from build123d import *
from build123d.topology import SkipClean

# Parameters (mm, degrees)
MAIN_ANGLE          = 180
CIRCULAR_BOSS_REACH = 111.487
SKETCH6_R           = 11.1125
CIRCULAR_CUT_DEPTH  = 110.4866698
SKETCH7_W           = 4.7625
SKETCH7_H           = 3.175
LPATTERN1_COUNT     = 3
LPATTERN1_PITCH     = 5.08


with BuildPart() as part:
    # Sketch1 → Main (revolve)
    with BuildSketch(Plane(origin=(0, 0, 0), x_dir=(0, 0, -1), z_dir=(1, 0, 0))):
        Polygon((38.1, 88.9), (0, 88.9), (0, 84.1375), (28.575, 84.1375), (28.575, 44.45), (34.925, 44.45), (34.925, 4.7625), (33.3375, 4.7625), (33.3375, 0), (38.1, 0), align=None)
    revolve(axis=Axis((0, 88.9, 0), (0, 1, 0)), revolution_arc=MAIN_ANGLE)

    # Sketch5 → Circular Boss (add, up to next)
    with BuildSketch(Plane.XY.offset(13.208), mode=Mode.PRIVATE) as circular_boss_sk1:
        with BuildLine():
            Line((0, 30.1625), (0, 58.7375))
            ThreePointArc((0, 58.7375), (-14.2875, 44.45), (0, 30.1625))
        make_face()
    circular_boss_tool1 = extrude(circular_boss_sk1.sketch, amount=CIRCULAR_BOSS_REACH, mode=Mode.PRIVATE) - part.part
    circular_boss = circular_boss_tool1.solids().sort_by_distance((-6.063803, 44.45, 13.208))[0]
    add(circular_boss)

    # Sketch6 → Circular Cut (cut, through all)
    with BuildSketch(Plane.XY.offset(13.208)):
        with Locations((0, 44.45)):
            Circle(SKETCH6_R)
    circular_cut = extrude(amount=CIRCULAR_CUT_DEPTH, mode=Mode.SUBTRACT)

    # Sketch7 → Cut-Revolve1 (revolve, cut)
    with BuildSketch(Plane(origin=(0, 7.447290845, 55.242674731), x_dir=(0, 0, -1), z_dir=(1, 0, 0))):
        with Locations((90.961424731, 63.990209155)):
            Rectangle(SKETCH7_W, SKETCH7_H)
    cut_revolve1 = revolve(axis=Axis((0, 73.025, 0), (0, -1, 0)), mode=Mode.SUBTRACT)

    # LPattern1: Cut-Revolve1 ×3
    with Locations(*[(0, i * LPATTERN1_PITCH, 0) for i in range(1, LPATTERN1_COUNT)]):
        add(cut_revolve1, mode=Mode.SUBTRACT)

    # Mirror1: Circular Boss, Circular Cut across plane
    add(circular_boss.mirror(Plane.XY))
    add(circular_cut.mirror(Plane.XY), mode=Mode.SUBTRACT)

    # Mirror2: part across face


with BuildPart() as part_1:
    with SkipClean():  # the faces are left unmerged after this step: merging them gives an invalid solid
        add(part.part)
        add(part.part.mirror(Plane(origin=(0, 74.450038597, 0), x_dir=(0, 0, 1), z_dir=(1, 0, 0))))


solid = part_1.part
The model under review builds one solid part; all positions refer to its coordinate system, in mm. A direction names the side the tool comes from. Coordinates: 2 decimals unless noted, no trailing zeros. Loops run counter-clockwise (first coordinate to the right, second up) from the corner with the lowest first, then second, coordinate; pieces in that order, holes last. Notation, with made-up numbers: (89, 80.5) -> (148, 80.5) arc R26 cw to (148, 114.5) -> close; hole circle Ø4 at (-28, 10.25). An arc over 180 degrees is marked (long way). Use a Markdown table: item, result. Add a question column.
1. To check wall thickness, follow line 1 (Y direction, x = 15.5, z = 32) (3 decimals); line 2 (X direction, y = 44, z = 20.5); line 3 (X direction, y = 44.5, z = 23). State the ranges of each line that lie inside material, in increasing order.
2. Add section B-B on z = 21. Give the number of separate pieces and of enclosed holes in the cut face, plus the area to 3 significant figures.
3. Machinability: for faces 1 (the face through (30, 44.45, 0)), 2 (the face through (9, 37, -13.208)), which of the approach directions +Z, -Z, +X, -X, +Y, -Y give a long, thin tool a straight path to every point of the face, cutting with its end or side? Answer none if there is none.
4. Clearance check with flat-ended pins moving along their axes: pin 1 Ø11.5 at (x, z) = (-12, 10) entering from -Y; pin 2 Ø3 at (x, y) = (10, 24) entering from -Z; pin 3 Ø7 at (x, y) = (-10.5, 51) entering from -Z; pin 4 Ø12 at (x, y) = (-3, 43.5) entering from +Z. State where each tip first meets the part, or that it passes through.
5. Add section A-A on y = 46. Write out the cut boundary in (x, z) (3 decimals).
Returned:
| question | item | result |
|---|---|---|
| 1 | line 1 | y = 0 to 69.85, 73.025 to 74.93, 78.105 to 80.01, 83.185 to 88.9 |
| 1 | line 2 | x = -32.11 to -28.28, -14.28 to -11.1, 11.1 to 14.28, 28.28 to 32.11 |
| 1 | line 3 | x = -30.37 to -16.96, -14.29 to -11.11, 11.11 to 14.29, 16.96 to 30.37 |
| 2 | separate pieces | 2 |
| 2 | enclosed holes | 1 |
| 2 | area | 1,790 mm² |
| 3 | face 1 | none |
| 3 | face 2 | -Y |
| 4 | pin 1 | stops at y = 32.13 |
| 4 | pin 2 | stops at z = -37.14 |
| 4 | pin 3 | stops at z = -37.37 |
| 4 | pin 4 | passes through |
| 5 | outline | (-14.203, -24.795) arc R28.575 cw to (-14.203, 24.795) -> (-14.203, 13.208) -> (-11.004, 13.208) -> (-11.004, 36.476) arc R38.1 ccw to (-11.004, -36.476) -> (-11.004, -13.208) -> (-14.203, -13.208) -> close; (11.004, -36.476) arc R38.1 ccw to (11.004, 36.476) -> (11.004, 13.208) -> (14.203, 13.208) -> (14.203, 24.795) arc R28.575 cw to (14.203, -24.795) -> (14.203, -13.208) -> (11.004, -13.208) -> close |
